Design review of the part built by this model. Coordinates are the model's own, in mm. A direction names the side the tool comes from. Coordinates: 2 decimals unless noted, no trailing zeros. Write each loop counter-clockwise with the first axis right and the second up, starting at its lowest first coordinate (ties: lowest second). Pieces come first, ordered by that corner, then holes.
```python
from build123d import *

# Parameters (mm, degrees)
F0_R         = 1.5
F1_DEPTH     = 4
F2_T1_DEPTH  = 15
F2_T3_DEPTH  = 120
F2_T5_DEPTH  = 7
F2_T7_DEPTH  = 10
F2_T9_DEPTH  = 16
F2_T11_DEPTH = 94
F2_T13_DEPTH = 16
F2_T15_DEPTH = 7
F2_T25_DEPTH = 12
F2_T29_DEPTH = 15
F2_T36_DEPTH = 15
F2_T40_DEPTH = 99
F2_T47_DEPTH = 99
F2_T51_DEPTH = 15
F2_T58_DEPTH = 15
F2_T62_DEPTH = 12


# Not quite as in the source:
# - a fillet or chamfer that OpenCascade refuses, or shapes differently, is made with other operations: its cross-section is extruded or revolved along the edge and cut away or added


with BuildPart() as f1:
    # F0 (on Front) → F1 (new body)
    with BuildSketch(Plane.XZ):
        Polygon((-55, 5), (-55, 0), (55, 0), (55, 5), (53, 5), (53, 10), (47, 10), (47, 5), (-47, 5), (-47, 10), (-53, 10), (-53, 5), align=None)
        with Locations((-50, 7.5)):
            Circle(F0_R, mode=Mode.SUBTRACT)
        with Locations((50, 7.5)):
            Circle(F0_R, mode=Mode.SUBTRACT)
    extrude(amount=F1_DEPTH)

    # F2: fillet of radius 2 on 14 edges, made by hand

    # F2_s2 → F2_t1 (cut)
    with BuildSketch(Plane.XY.offset(-5)):
        with BuildLine():
            ThreePointArc((-55, -2), (-54.4142135624, -3.4142135624), (-53, -4))
            Line((-53, -4), (-55, -4))
            Line((-55, -4), (-55, -2))
        make_face()
        with BuildLine():
            ThreePointArc((55, -2), (54.4142135624, -3.4142135624), (53, -4))
            Line((53, -4), (55, -4))
            Line((55, -4), (55, -2))
        make_face()
    extrude(amount=F2_T1_DEPTH, mode=Mode.SUBTRACT)

    # F2_s4 → F2_t3 (cut)
    with BuildSketch(Plane.YZ.offset(-60)):
        with BuildLine():
            ThreePointArc((-2, 0), (-3.4142135624, 0.5857864376), (-4, 2))
            Line((-4, 2), (-4, 0))
            Line((-4, 0), (-2, 0))
        make_face()
    extrude(amount=F2_T3_DEPTH, mode=Mode.SUBTRACT)

    # F2_s6 → F2_t5 (cut)
    with BuildSketch(Plane.YZ.offset(53)):
        with BuildLine():
            ThreePointArc((-2, 5), (-3.4142135624, 4.4142135624), (-4, 3))
            Line((-4, 3), (-4, 5))
            Line((-4, 5), (-2, 5))
        make_face()
    extrude(amount=F2_T5_DEPTH, mode=Mode.SUBTRACT)

    # F2_s8 → F2_t7 (cut)
    with BuildSketch(Plane.XY.offset(5)):
        with BuildLine():
            ThreePointArc((53, -2), (52.4142135624, -3.4142135624), (51, -4))
            Line((51, -4), (53, -4))
            Line((53, -4), (53, -2))
        make_face()
        with BuildLine():
            ThreePointArc((47, -2), (47.5857864376, -3.4142135624), (49, -4))
            Line((49, -4), (47, -4))
            Line((47, -4), (47, -2))
        make_face()
        with BuildLine():
            ThreePointArc((-47, -2), (-47.5857864376, -3.4142135624), (-49, -4))
            Line((-49, -4), (-47, -4))
            Line((-47, -4), (-47, -2))
        make_face()
        with BuildLine():
            ThreePointArc((-53, -2), (-52.4142135624, -3.4142135624), (-51, -4))
            Line((-51, -4), (-53, -4))
            Line((-53, -4), (-53, -2))
        make_face()
    extrude(amount=F2_T7_DEPTH, mode=Mode.SUBTRACT)

    # F2_s10 → F2_t9 (cut)
    with BuildSketch(Plane.YZ.offset(42)):
        with BuildLine():
            ThreePointArc((-2, 10), (-3.4142135624, 9.4142135624), (-4, 8))
            Line((-4, 8), (-4, 10))
            Line((-4, 10), (-2, 10))
        make_face()
    extrude(amount=F2_T9_DEPTH, mode=Mode.SUBTRACT)

    # F2_s12 → F2_t11 (cut)
    with BuildSketch(Plane.YZ.offset(-47)):
        with BuildLine():
            ThreePointArc((-2, 5), (-3.4142135624, 4.4142135624), (-4, 3))
            Line((-4, 3), (-4, 5))
            Line((-4, 5), (-2, 5))
        make_face()
    extrude(amount=F2_T11_DEPTH, mode=Mode.SUBTRACT)

    # F2_s14 → F2_t13 (cut)
    with BuildSketch(Plane.YZ.offset(-58)):
        with BuildLine():
            ThreePointArc((-2, 10), (-3.4142135624, 9.4142135624), (-4, 8))
            Line((-4, 8), (-4, 10))
            Line((-4, 10), (-2, 10))
        make_face()
    extrude(amount=F2_T13_DEPTH, mode=Mode.SUBTRACT)

    # F2_s16 → F2_t15 (cut)
    with BuildSketch(Plane.YZ.offset(-60)):
        with BuildLine():
            ThreePointArc((-2, 5), (-3.4142135624, 4.4142135624), (-4, 3))
            Line((-4, 3), (-4, 5))
            Line((-4, 5), (-2, 5))
        make_face()
    extrude(amount=F2_T15_DEPTH, mode=Mode.SUBTRACT)

    # F2_s17 → F2_t18 (revolve, cut)
    with BuildSketch(Plane.XY.offset(7.5)):
        with BuildLine():
            ThreePointArc((-48.5, -2), (-47.9142135624, -3.4142135624), (-46.5, -4))
            Line((-46.5, -4), (-48.5, -4))
            Line((-48.5, -4), (-48.5, -2))
        make_face()
    revolve(axis=Axis((-50, -4, 7.5), (0, -1, 0)), mode=Mode.SUBTRACT)

    # F2_s19 → F2_t20 (revolve, cut)
    with BuildSketch(Plane.XY.offset(7.5)):
        with BuildLine():
            ThreePointArc((51.5, -2), (52.0857864376, -3.4142135624), (53.5, -4))
            Line((53.5, -4), (51.5, -4))
            Line((51.5, -4), (51.5, -2))
        make_face()
    revolve(axis=Axis((50, -4, 7.5), (0, -1, 0)), mode=Mode.SUBTRACT)


with BuildPart() as f2_tool23:
    # F2_s24 → F2_t25 (new body)
    with BuildSketch(Plane.YZ.offset(60)):
        with BuildLine():
            ThreePointArc((-2, 5), (-3.4142135624, 4.4142135624), (-4, 3))
            Line((-4, 3), (-4, 5))
            Line((-4, 5), (-2, 5))
        make_face()
    extrude(amount=-F2_T25_DEPTH)

    split(bisect_by=Plane.YZ.offset(53), keep=Keep.BOTTOM)


with BuildPart() as f2_tool27:
    # F2_s28 → F2_t29 (new body)
    with BuildSketch(Plane.XY):
        with BuildLine():
            ThreePointArc((53, -2), (52.4142135624, -3.4142135624), (51, -4))
            Line((51, -4), (53, -4))
            Line((53, -4), (53, -2))
        make_face()
    extrude(amount=F2_T29_DEPTH)

    split(bisect_by=Plane.XY.offset(5), keep=Keep.BOTTOM)


with BuildPart() as f2_tool23_1:
    add(f2_tool23.part)

    # F2_t31: intersect F2_tool27
    add(f2_tool27.part, mode=Mode.INTERSECT)


with BuildPart() as f1_1:
    add(f1.part)

    # F2_t21: cut F2_tool23
    add(f2_tool23_1.part, mode=Mode.SUBTRACT)


with BuildPart() as f2_tool34:
    # F2_s35 → F2_t36 (new body)
    with BuildSketch(Plane.XY.offset(15)):
        with BuildLine():
            ThreePointArc((47, -2), (47.5857864376, -3.4142135624), (49, -4))
            Line((49, -4), (47, -4))
            Line((47, -4), (47, -2))
        make_face()
    extrude(amount=-F2_T36_DEPTH)

    split(bisect_by=Plane.XY.offset(5), keep=Keep.BOTTOM)


with BuildPart() as f2_tool38:
    # F2_s39 → F2_t40 (new body)
    with BuildSketch(Plane.YZ.offset(52)):
        with BuildLine():
            ThreePointArc((-2, 5), (-3.4142135624, 4.4142135624), (-4, 3))
            Line((-4, 3), (-4, 5))
            Line((-4, 5), (-2, 5))
        make_face()
    extrude(amount=-F2_T40_DEPTH)

    split(bisect_by=Plane.YZ.offset(47), keep=Keep.TOP)


with BuildPart() as f2_tool34_1:
    add(f2_tool34.part)

    # F2_t42: intersect F2_tool38
    add(f2_tool38.part, mode=Mode.INTERSECT)


with BuildPart() as f1_2:
    add(f1_1.part)

    # F2_t32: cut F2_tool34
    add(f2_tool34_1.part, mode=Mode.SUBTRACT)


with BuildPart() as f2_tool45:
    # F2_s46 → F2_t47 (new body)
    with BuildSketch(Plane.YZ.offset(47)):
        with BuildLine():
            ThreePointArc((-2, 5), (-3.4142135624, 4.4142135624), (-4, 3))
            Line((-4, 3), (-4, 5))
            Line((-4, 5), (-2, 5))
        make_face()
    extrude(amount=-F2_T47_DEPTH)

    split(bisect_by=Plane.YZ.offset(-47), keep=Keep.BOTTOM)


with BuildPart() as f2_tool49:
    # F2_s50 → F2_t51 (new body)
    with BuildSketch(Plane.XY):
        with BuildLine():
            ThreePointArc((-47, -2), (-47.5857864376, -3.4142135624), (-49, -4))
            Line((-49, -4), (-47, -4))
            Line((-47, -4), (-47, -2))
        make_face()
    extrude(amount=F2_T51_DEPTH)

    split(bisect_by=Plane.XY.offset(5), keep=Keep.BOTTOM)


with BuildPart() as f2_tool45_1:
    add(f2_tool45.part)

    # F2_t53: intersect F2_tool49
    add(f2_tool49.part, mode=Mode.INTERSECT)


with BuildPart() as f1_3:
    add(f1_2.part)

    # F2_t43: cut F2_tool45
    add(f2_tool45_1.part, mode=Mode.SUBTRACT)


with BuildPart() as f2_tool56:
    # F2_s57 → F2_t58 (new body)
    with BuildSketch(Plane.XY.offset(15)):
        with BuildLine():
            ThreePointArc((-53, -2), (-52.4142135624, -3.4142135624), (-51, -4))
            Line((-51, -4), (-53, -4))
            Line((-53, -4), (-53, -2))
        make_face()
    extrude(amount=-F2_T58_DEPTH)

    split(bisect_by=Plane.XY.offset(5), keep=Keep.BOTTOM)


with BuildPart() as f2_tool60:
    # F2_s61 → F2_t62 (new body)
    with BuildSketch(Plane.YZ.offset(-48)):
        with BuildLine():
            ThreePointArc((-2, 5), (-3.4142135624, 4.4142135624), (-4, 3))
            Line((-4, 3), (-4, 5))
            Line((-4, 5), (-2, 5))
        make_face()
    extrude(amount=-F2_T62_DEPTH)

    split(bisect_by=Plane.YZ.offset(-53), keep=Keep.TOP)


with BuildPart() as f2_tool56_1:
    add(f2_tool56.part)

    # F2_t64: intersect F2_tool60
    add(f2_tool60.part, mode=Mode.INTERSECT)


with BuildPart() as f1_4:
    add(f1_3.part)

    # F2_t54: cut F2_tool56
    add(f2_tool56_1.part, mode=Mode.SUBTRACT)


solid = f1_4.part
```
(1) Wall thickness on line 1 (X direction, y = -1, z = 7.75); line 2 (Z direction, x = -50, y = -0.9); line 3 (X direction, y = -3.55, z = 4.75): over which ranges is each line inside the solid? List them lowest first.
(2) Insertion check: pin 1 Ø1 at (x, y) = (-54, -0.5) entering from +Z; pin 2 Ø1.6 at (y, z) = (-1.5, 8) entering from -X; pin 3 Ø1.6 at (y, z) = (-1, 8) entering from +X. Each pin has a flat end and moves straight along its axis. Give the tip position at first contact, or say it passes through.
(3) Consider section C-C (z = 1). Give the boundary of the cut face in (x, y), plus the area to 3 significant figures.
(4) Consider section A-A (z = 7.5). Give the boundary of the cut face in (x, y), plus the area to 3 significant figures.
(5) Consider section B-B (x = 44). Give the boundary of the cut face in (y, z).
(6) For faces 4 (the cylindrical face through (-0.69, -3.4, 4.43)), 5 (the flat face through (-47, -1, 7)), 6 (the flat face through (-53, -1, 8)), list the 3-axis set-ups (+Z, -Z, +X, -X, +Y, -Y) from which the entire face can be reached by the end or side of a thin tool; tool diameter is ignored.
(7) Consider section D-D (x = -50). Give the boundary of the cut face in (y, z), plus the area to 3 significant figures.
(8) Mouldability with a two-part tool opening along X and no side actions: class faces 1 (the cylindrical face through (-52.65, -3.13, 6.45)), 2 (the flat face through (1, -1, 5)), 3 (the cylindrical face through (-0.77, -3.4, 0.57)) as +X half, -X half, draft (parallel to the pull), parting line (faces both ways), or undercut.
Results:
1. line 1: x = -53 to -51.48, -48.52 to -47, 47 to 48.52, 51.48 to 53
1. line 2: z = 0 to 6, 9 to 10
1. line 3: x = -52.26 to -47.74, 47.74 to 52.26
2. pin 1: stops at z = 5
2. pin 2: stops at x = -53
2. pin 3: stops at x = 53
3. outline: (-55, -2) arc R2 ccw to (-54, -3.73) - (54, -3.73) arc R2 ccw to (55, -2) - (55, 0) - (-55, 0) - close
3. area: 410 mm2
4. outline: (-53, -2) arc R2 ccw to (-52.25, -3.56) arc R2 ccw to (-51.5, -2) - (-51.5, 0) - (-53, 0) - close; (-48.5, -2) arc R2 ccw to (-47.75, -3.56) arc R2 ccw to (-47, -2) - (-47, 0) - (-48.5, 0) - close; (47, -2) arc R2 ccw to (47.75, -3.56) arc R2 ccw to (48.5, -2) - (48.5, 0) - (47, 0) - close; (51.5, -2) arc R2 ccw to (52.25, -3.56) arc R2 ccw to (53, -2) - (53, 0) - (51.5, 0) - close
4. area: 18.5 mm2
5. outline: (-4, 2) arc R2 ccw to (-2, 0) - (0, 0) - (0, 5) - (-2, 5) arc R2 ccw to (-4, 3) - close
6. face 4: +Z, -Y
6. face 5: +Z, +Y, -Y
6. face 6: +Z, -X, +Y, -Y
7. outline: (-4, 2) arc R2 ccw to (-2, 0) - (0, 0) - (0, 6) - (-2, 6) arc R2 ccw to (-4, 4) - close; (-3.32, 9.5) arc R2 ccw to (-2, 9) - (0, 9) - (0, 10) - (-2, 10) arc R2 ccw to start
7. area: 25.2 mm2
8. face 1: -X half
8. face 2: undercut
8. face 3: draft
